The listing builds one solid part. Answer for the finished solid, in the listing's coordinates (mm). A direction names the side the tool comes from. Coordinates: 2 decimals unless noted, no trailing zeros. Loops run counter-clockwise (first coordinate to the right, second up) from the corner with the lowest first, then second, coordinate; pieces in that order, holes last. Notation, with made-up numbers: (-19, -37) - (6, -37) arc R24 cw to (6, -1) - close; hole circle Ø11 at (-29, 62). An arc over 180 degrees is marked (long way). One line per question, with ' | ' between items.
from build123d import *

# Parameters (mm, degrees)
CUT_EXTRUDE1_START = -2
CUT_EXTRUDE1_DEPTH = 2
SKETCH4_R          = 1.732050808
CUT_EXTRUDE2_DEPTH = 0.5
CUT_EXTRUDE2_TAPER = 45


with BuildPart() as part:
    # Sketch2 → Revolve1 (revolve)
    with BuildSketch(Plane(origin=(0, 0, 0), x_dir=(0, 0, -1), z_dir=(1, 0, 0))):
        Polygon((-4.3, 3.5), (-0.7, 3.5), (-0.5, 3.3), (-0.5, 2), (3.8, 2), (4.5, 1.3), (4.5, 0), (-4.5, 0), (-4.5, 3.3), align=None)
    revolve(axis=Axis((0, 0, -4.5), (0, 0, 1)))

    # Sketch3 → Cut-Extrude1 (cut)
    with BuildSketch(Plane.XY.offset(4.5).offset(CUT_EXTRUDE1_START)):
        Polygon((0, 1.732050808), (-1.5, 0.866025404), (-1.5, -0.866025404), (0, -1.732050808), (1.5, -0.866025404), (1.5, 0.866025404), align=None)
    extrude(amount=CUT_EXTRUDE1_DEPTH, mode=Mode.SUBTRACT)

    # Sketch4 → Cut-Extrude2 (cut)
    with BuildSketch(Plane.XY.offset(4.5)):
        Circle(SKETCH4_R)
    extrude(amount=-CUT_EXTRUDE2_DEPTH, taper=CUT_EXTRUDE2_TAPER, mode=Mode.SUBTRACT)


solid = part.part
Item 1: The mould has two halves that part along X. Classify faces 4 (the face through (1.341, 3.233, 2.475)), 5 (the face through (1.4, -1.4, 4.5)), 6 (the face through (-0.8, 1.4, 4.38)): pulls with the +X half, pulls with the -X half, needs draft (parallel to the pull), parting line crosses it, or undercut.
Taken from the geometry:
face 4: parting line crosses it | face 5: needs draft | face 6: undercut
Item 2: Which of the six approach directions +Z, -Z, +X, -X, +Y, -Y give full straight-line access (tool end or side, diameter ignored) to faces 1 (the face through (-0.74, 1.305, 3.486)), 2 (the face through (2.2, 0, 0.5)), 3 (the face through (0, 0, -4.5))?
Taken from the geometry:
face 1: +Z | face 2: -Z | face 3: -Z, +X, -X, +Y, -Y
Item 3: Find section B-B, the plane z = -1. Write down the section's boundary in (x, y).
Taken from the geometry:
outline: circle Ø4 at (0, 0)
Item 4: Find section A-A, the plane z = 1.75. Write down the section's boundary in (x, y).
Taken from the geometry:
outline: circle Ø7 at (0, 0)
Item 5: Each of these flat-tipped pins is pushed along its axis until it touches: pin 1 Ø0.9 at (x, y) = (0.5, 0.5) entering from +Z; pin 2 Ø1 at (x, z) = (2, 3.5) entering from +Y; pin 3 Ø4 at (y, z) = (-0.5, -3) entering from -X. Where does it stop, or does it pass through?
Taken from the geometry:
pin 1: stops at z = 2.5 | pin 2: stops at y = 3.16 | pin 3: stops at x = -2
Item 6: Find the intervals of material crossed by line 1 (Z direction, x = 2.5, y = 0); line 2 (Z direction, x = 0.25, y = 0.75); line 3 (Y direction, x = -1, z = 3), in increasing order. Write a range as [from, to].
Taken from the geometry:
line 1: z = [0.5, 4.5] | line 2: z = [-4.5, 2.5] | line 3: y = [-3.35, -1.15], [1.15, 3.35]
